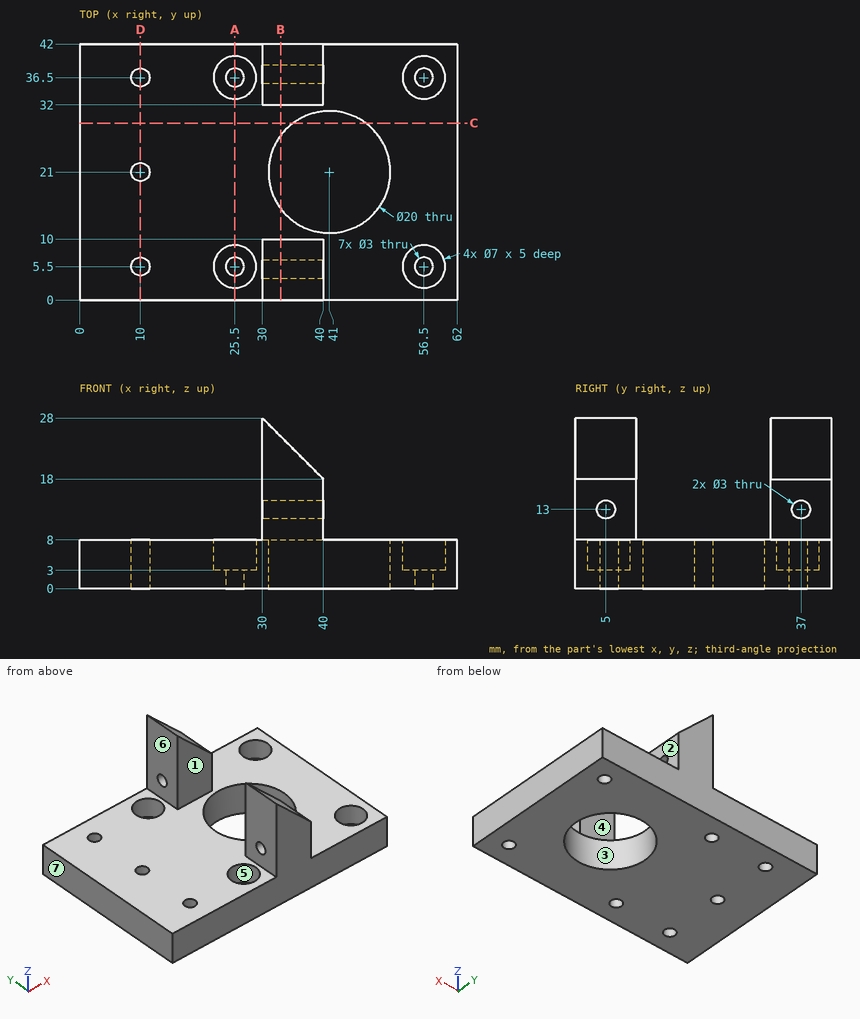
Design review of the part shown in the three views and the two pictorial views. Dimensions are in mm from the part's minimum x, y and z. A direction names the side the tool comes from. Coordinates: 2 decimals unless noted, no trailing zeros. Loops run counter-clockwise (first coordinate to the right, second up) from the corner with the lowest first, then second, coordinate; pieces in that order, holes last. Notation, with made-up numbers: M 7.5,60 L 27.5,60 A10 ccw 27.5,68 Z; hole C 7.5,-19.75 d6. An arc over 180 degrees is marked long. One line per question, with ' | ' between items.
(1) Draft analysis for pull direction X (two halves, no side actions). For the marked faces 1, 2 and 3, state which applies: released by +X, released by -X, zero draft, split by the parting line, or undercut.
Filled in:
face 1: zero draft | face 2: released by +X | face 3: undercut
(2) Wall thickness on probe 1 along Y at (x, z) = (25.5, 0.95); probe 2 along Y at (x, z) = (10, 3); probe 3 along Y at (x, z) = (56.5, 4.6): over which ranges is each line inside the solid? List them lowest first.
Filled in:
probe 1: y = 0 to 4, 7 to 35, 38 to 42 | probe 2: y = 0 to 4, 7 to 19.5, 22.5 to 35, 38 to 42 | probe 3: y = 0 to 2, 9 to 33, 40 to 42
(3) Machinability: for the marked faces 4, 5, 6 and 7, which of the approach directions +Z, -Z, +X, -X, +Y, -Y give a long, thin tool a straight path to every point of the face, cutting with its end or side? Answer none if there is none.
Filled in:
face 4: +Z, +X, -X | face 5: +Z | face 6: +Z, -X, +Y, -Y | face 7: +Z, -Z, -X, +Y, -Y
(4) We need section B-B (x = 33). Give the boundary of the cut face in (y, z), and give its area (3 significant figures).
Filled in:
outline: M 0,0 L 15,0 L 15,8 L 10,8 L 10,25 L 0,25 Z; M 27,0 L 42,0 L 42,25 L 32,25 L 32,8 L 27,8 Z; hole C 5,13 d3; hole C 37,13 d3 | area: 566 mm^2
(5) We need section C-C (y = 29). Give the boundary of the cut face in (x, z).
Filled in:
outline: M 0,0 L 35,0 L 35,8 L 0,8 Z; M 47,0 L 62,0 L 62,8 L 47,8 Z
(6) For pin 1 Ø4 at (y, z) = (37, 13) entering from -X; pin 2 Ø8 at (y, z) = (33.5, 18) entering from +X; pin 3 Ø4 at (x, y) = (56.5, 5.5) entering from +Z; pin 4 Ø4 at (x, y) = (29.5, 22.5) entering from -Z, all flat-tipped, find the tip position at first contact; note any pin that passes through.
Filled in:
pin 1: stops at x = 30 | pin 2: stops at x = 40 | pin 3: stops at z = 3 | pin 4: stops at z = 0
(7) We need section A-A (x = 25.5). Give the boundary of the cut face in (y, z), and give its area (3 significant figures).
Filled in:
outline: M 0,0 L 4,0 L 4,3 L 2,3 L 2,8 L 0,8 Z; M 7,0 L 35,0 L 35,3 L 33,3 L 33,8 L 9,8 L 9,3 L 7,3 Z; M 38,0 L 42,0 L 42,8 L 40,8 L 40,3 L 38,3 Z | area: 248 mm^2
(8) We need section D-D (x = 10). Give the boundary of the cut face in (y, z), and give its area (3 significant figures).
Filled in:
outline: M 0,0 L 4,0 L 4,8 L 0,8 Z; M 7,0 L 19.5,0 L 19.5,8 L 7,8 Z; M 22.5,0 L 35,0 L 35,8 L 22.5,8 Z; M 38,0 L 42,0 L 42,8 L 38,8 Z | area: 264 mm^2
